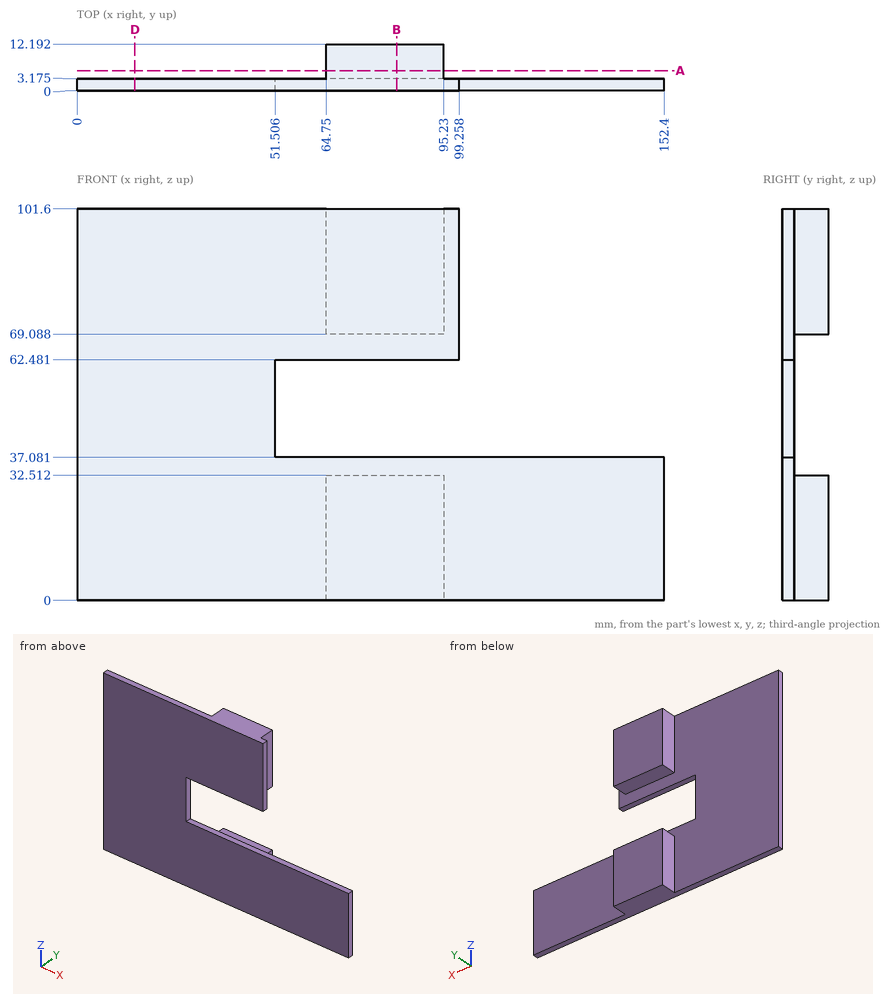
Answer from the drawing. Dimensions are ordinates in mm from the lowest x, y and z of the part. Coordinates: 2 decimals unless noted, no trailing zeros. Order: outer loops, then holes, each group sorted by start corner. A loop starts at its lowest first (then second) coordinate and runs counter-clockwise, first axis right, second up. Notation, with made-up numbers: (-20.5, -15.75) -> (-10.5, -15.75) arc R23 cw to (-10.5, -5.75) -> close; hole circle Ø3 at (-15, 58.25). An arc over 180 degrees is marked (long way). Answer as a JSON object with one key per item and string values.
1) A cutting plane is placed at B-B, the plane x = 83. Determine the outline of the cut face in (y, z) (1 decimal).
Model answer:
{"outline": "(0, 0) -> (12.2, 0) -> (12.2, 32.5) -> (3.2, 32.5) -> (3.2, 37.1) -> (0, 37.1) -> close; (0, 62.5) -> (3.2, 62.5) -> (3.2, 69.1) -> (12.2, 69.1) -> (12.2, 101.6) -> (0, 101.6) -> close"}
2) Consider line 1 along Z through (x, y) = (66.5, 2.5); line 2 along X through (y, z) = (9.5, 76.5); line 3 along Z through (x, y) = (94, 11.25). Determine where each line is inside the solid, lowest interval first. Write a range as from..to.
Model answer:
{"line 1": "z = 0..37.08, 62.48..101.6", "line 2": "x = 64.75..95.23", "line 3": "z = 0..32.51, 69.09..101.6"}
3) Each of these flat-tipped pins is pushed along its axis until it touches: pin 1 (4 mm diameter, centred on x = 117, y = 7, fed in from +Z) (3 decimals); pin 2 (1.6 mm diameter, centred on y = 1, z = 53.5, fed in from +X); pin 3 (1 mm diameter, centred on y = 2, z = 91.5, fed in from +X); pin 4 (2.5 mm diameter, centred on y = 8, z = 24, fed in from +X). Where does it stop, or does it pass through?
Model answer:
{"pin 1": "passes through", "pin 2": "stops at x = 51.51", "pin 3": "stops at x = 99.26", "pin 4": "stops at x = 95.23"}
4) A cutting plane is placed at D-D, the plane x = 15. Determine the outline of the cut face in (y, z) (1 decimal).
Model answer:
{"outline": "(0, 0) -> (3.2, 0) -> (3.2, 101.6) -> (0, 101.6) -> close"}
5) A cutting plane is placed at A-A, the plane y = 5.25. Determine the outline of the cut face in (x, z), plus the area to 3 significant figures.
Model answer:
{"outline": "(64.75, 0) -> (95.23, 0) -> (95.23, 32.51) -> (64.75, 32.51) -> close; (64.75, 69.09) -> (95.23, 69.09) -> (95.23, 101.6) -> (64.75, 101.6) -> close", "area": "1,980 mm²"}
